Verification items for the finished model (mm, model axes). Face numbers are marked on the shaded views. Coordinates: 2 decimals unless noted, no trailing zeros. Write each loop counter-clockwise with the first axis right and the second up, starting at its lowest first coordinate (ties: lowest second). Pieces come first, ordered by that corner, then holes. Notation, with made-up numbers: M -32,-7 L 26,-7 A28 ccw 26,27 Z; hole C 86.25,-40 d6. An arc over 180 degrees is marked long. Answer in a Markdown table with one row per item.
from build123d import *

# Parameters (mm, degrees)
F0_R     = 16
F0_R_2   = 4.9
F1_DEPTH = 5
F2_R     = 1.75
F3_DEPTH = 25


with BuildPart() as f1:
    # F0 (on Top) → F1 (new body)
    with BuildSketch(Plane.XY):
        Circle(F0_R)
        Circle(F0_R_2, mode=Mode.SUBTRACT)
    extrude(amount=F1_DEPTH)

    # F2 (on face) → F3 (cut)
    with BuildSketch(Plane.XY.offset(5)):
        with Locations((0, 12.5)):
            Circle(F2_R)
        with Locations((10.825318, 6.25)):
            Circle(F2_R)
        with Locations((10.825318, -6.25)):
            Circle(F2_R)
        with Locations((0, -12.5)):
            Circle(F2_R)
        with Locations((-10.825318, -6.25)):
            Circle(F2_R)
        with Locations((-10.825318, 6.25)):
            Circle(F2_R)
    extrude(amount=-F3_DEPTH, mode=Mode.SUBTRACT)


solid = f1.part
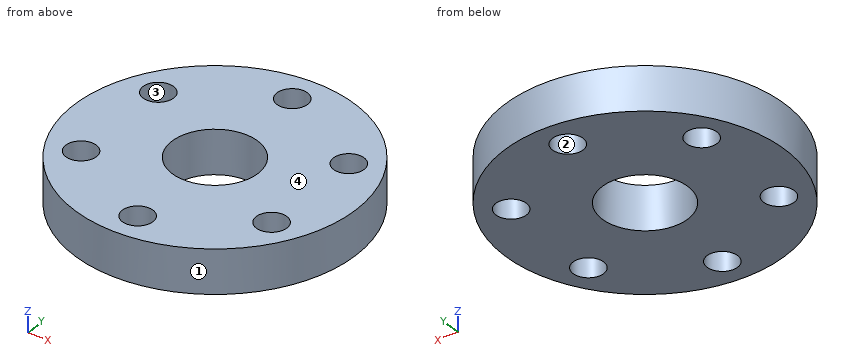
1) Release check for a two-part mould opening along X. For the marked faces 1, 2, 3 and 4 record: +X half, -X half, draft (parallel to the pull), parting line (faces both ways), or undercut.
Response values:
| item | result |
|---|---|
| face 1 | parting line |
| face 2 | undercut |
| face 3 | undercut |
| face 4 | draft |
2) Sectioned sample at B-B (z = 3.55). Record the cut outline in (x, y).
Response values:
| item | result |
|---|---|
| outline | C 0,0 d32; hole C -10.83,-6.25 d3.5; hole C -10.83,6.25 d3.5; hole C 0,0 d9.8; hole C 0,-12.5 d3.5; hole C 0,12.5 d3.5; hole C 10.83,-6.25 d3.5; hole C 10.83,6.25 d3.5 |
3) Sectioned sample at D-D (y = 7). Record the cut outline in (x, z).
Response values:
| item | result |
|---|---|
| outline | M -14.39,0 L -12.41,0 L -12.41,5 L -14.39,5 Z; M -9.24,0 L 9.24,0 L 9.24,5 L -9.24,5 Z; M 12.41,0 L 14.39,0 L 14.39,5 L 12.41,5 Z |
4) Sectioned sample at A-A (y = 0). Record the cut outline in (x, z), then the cut area to 3 significant figures.
Response values:
| item | result |
|---|---|
| outline | M -16,0 L -4.9,0 L -4.9,5 L -16,5 Z; M 4.9,0 L 16,0 L 16,5 L 4.9,5 Z |
| area | 111 mm² |
5) Thickness scan on L1, parallel to Y at x = 0, z = 3.95; L2, parallel to Y at x = -12, z = 4.3; L3, parallel to X at y = -7.5, z = 1.65. Record the ranges inside material, lowest first. Write a range as [from, to].
Response values:
| item | result |
|---|---|
| L1 | y = [-16, -14.25], [-10.75, -4.9], [4.9, 10.75], [14.25, 16] |
| L2 | y = [-10.58, -7.55], [-4.95, 4.95], [7.55, 10.58] |
| L3 | x = [-14.13, -12.05], [-9.6, 9.6], [12.05, 14.13] |
6) Depth check by flat-ended pin: pin 1 (4 mm diameter, centred on x = 10.83, y = 6.25, fed in from -Z); pin 2 (1.5 mm diameter, centred on x = -5, z = 2.5, fed in from -Y); pin 3 (1 mm diameter, centred on x = 9, z = 2, fed in from -Y); pin 4 (3 mm diameter, centred on y = -11, z = 3, fed in from +X). Enter the tip coordinate at first touch or a pass-through.
Response values:
| item | result |
|---|---|
| pin 1 | stops at z = 0 |
| pin 2 | stops at y = -15.43 |
| pin 3 | stops at y = -13.56 |
| pin 4 | stops at x = 12.87 |
7) Sectioned sample at C-C (x = 0). Record the cut outline in (y, z), then the cut area to 3 significant figures.
Response values:
| item | result |
|---|---|
| outline | M -16,0 L -14.25,0 L -14.25,5 L -16,5 Z; M -10.75,0 L -4.9,0 L -4.9,5 L -10.75,5 Z; M 4.9,0 L 10.75,0 L 10.75,5 L 4.9,5 Z; M 14.25,0 L 16,0 L 16,5 L 14.25,5 Z |
| area | 76.0 mm² |
